Geometry check sheet. Reference: the model listing, model coordinates, mm. Face numbers are marked on the shaded views. A direction names the side the tool comes from. Give positions to 0.01 mm unless a question says otherwise; leave off trailing zeros. Write each loop counter-clockwise with the first axis right and the second up, starting at its lowest first coordinate (ties: lowest second). Pieces come first, ordered by that corner, then holes. Notation, with made-up numbers: (21.25, 82.25) -> (55.25, 82.25) arc R30 cw to (55.25, 113.25) -> close; hole circle Ø2 at (88.5, 82). An arc over 180 degrees is marked (long way). Write item = value, one per line. Start each with the question number.
1. Depth check by flat-ended pin: P1, Ø3, axis at x = -1, z = 14, coming from the +Y side; P2, Ø8, axis at y = 6.5, z = 1.5, coming from the +X side; P3, Ø1.2, axis at x = -0.5, z = -14.5, coming from the -Y side. Enter the tip coordinate at first touch or a pass-through.
2. Cross-section at B-B, the plane y = -19.5. Record the cut outline in (x, z).
3. Cross-section at C-C, the plane z = 14. Record the cut outline in (x, y), plus the area to 3 significant figures.
4. Cross-section at A-A, the plane y = 8. Record the cut outline in (x, z), plus the area to 3 significant figures.
5. Cross-section at D-D, the plane y = 13. Record the cut outline in (x, z).
6. Thickness scan on line 1 along Z through (x, y) = (-1, -19); line 2 along X through (y, z) = (-20.7, -14); line 3 along X through (y, z) = (13, -24). Record the ranges inside material, lowest first.
7. Set-up check for the marked faces 5, 6 and 7: record each of +Z, -Z, +X, -X, +Y, -Y from which the full face is reachable in a straight line by a thin tool's end or side.
8. Mould release check, pull along Z, two halves, no side actions. Record for the marked faces 1, 2, 3 and 4: pulls with the +Z half, pulls with the -Z half, needs draft (parallel to the pull), parting line crosses it, or undercut.
Solid Edge part; units mm, degrees
sketch "Sketch1" plane through (0, 0, 0) normal (1, 0, 0) x (0, 1, 0)
  line L0 (-23.5, -27) -> (23.5, -27)
  line L1 (23.5, -27) -> (23.5, 27)
  line L2 (23.5, 27) -> (-23.5, 27)
  line L3 (-23.5, 27) -> (-23.5, -27)
  dimension "D1" = 23.5
  dimension "D2" = 23.5
extrude "Protrusion1" add sketch "Sketch1" along normal mid plane 12
hole "Bohrung_1" at (-1, -23.5, 14) direction (0, 1, 0) diameter 4 depth 6
hole "Hole1" at (-1, -23.5, -14) direction (0, 1, 0) diameter 4 depth 6
sketch "Sketch2" plane through (6, 0, 0) normal (1, 0, 0) x (0, 1, 0)
  line L0 (23.5, -4) -> (10, 13)
  line L1 (10, 13) -> (10, 3)
  line L2 (10, 3) -> (2.5, 3)
  line L3 (2.5, 3) -> (2.5, 18)
  line L4 (2.5, 18) -> (23.5, 18)
  line L5 (23.5, 18) -> (23.5, -4)
  dimension "D1" = 2.5
  dimension "D2" = 10
  dimension "D3" = 2.5
  dimension "D4" = 10
extrude "Extrusionsausschnitt_1" cut sketch "Sketch2" against normal blind 135.5146
sketch "Sketch3" plane through (6, 0, 0) normal (1, 0, 0) x (0, 1, 0)
  spline S0 degree 3 poles (12.1174, 10.3337) (10.891, 11.9811) (10.2801, 12.3852) (10, 11.2459) knots 0 0 0 0 1 1 1 1
  line L0 (9.0244, 13.5703) -> (10, 11.2459)
  line L1 (12.1174, 14.0202) -> (9.0244, 13.5703)
  line L2 (12.1174, 10.3337) -> (12.1174, 14.0202)
extrude "Extrusionsausschnitt_3" cut sketch "Sketch3" along normal mid plane 89.7467
fillet "Verrundung_1" radius 10 1 edges at (0, 23.5, -4)
sketch "Sketch4" plane through (6, 0, 0) normal (1, 0, 0) x (0, 1, 0)
  line L0 (-23.5, -27) -> (23.5, -27)
  line L1 (23.5, -27) -> (23.5, -25)
  line L2 (23.5, -25) -> (-23.5, -25)
  line L3 (-23.5, -25) -> (-23.5, -27)
  dimension "D1" = 23.5
extrude "Extrusionsausprägung_5" add sketch "Sketch4" along normal blind 2
properties part number "40" material "Polyacticacid"
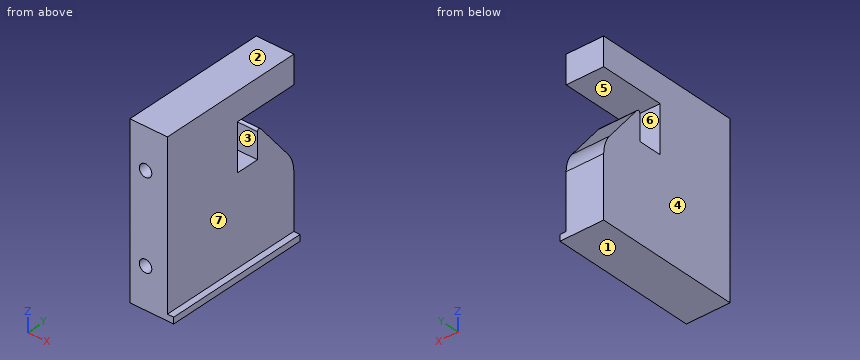
Answers:
q1.P1 = 2.5
q1.P2 = 6
q1.P3 = -17.5
q2.outline = (-6, -27) -> (8, -27) -> (8, -25) -> (6, -25) -> (6, 27) -> (-6, 27) -> close; hole circle Ø4 at (-1, -14); hole circle Ø4 at (-1, 14)
q3.outline = (-6, -23.5) -> (-3, -23.5) -> (-3, -17.5) -> (1, -17.5) -> (1, -23.5) -> (6, -23.5) -> (6, 2.5) -> (-6, 2.5) -> close
q3.area = 288 mm^2
q4.outline = (-6, -27) -> (8, -27) -> (8, -25) -> (6, -25) -> (6, 3) -> (-6, 3) -> close; (-6, 18) -> (6, 18) -> (6, 27) -> (-6, 27) -> close
q4.area = 472 mm^2
q5.outline = (-6, -27) -> (8, -27) -> (8, -25) -> (6, -25) -> (6, 9.22) -> (-6, 9.22) -> close; (-6, 18) -> (6, 18) -> (6, 27) -> (-6, 27) -> close
q6.line_1 = -27 to -16, -12 to 12, 16 to 27
q6.line_2 = -6 to -3, 1 to 6
q6.line_3 = -6 to 6
q7.face_5 = +X, -X, +Y
q7.face_6 = +X, -X
q7.face_7 = +Z, +X, +Y, -Y
q8.face_1 = pulls with the -Z half
q8.face_2 = pulls with the +Z half
q8.face_3 = undercut
q8.face_4 = needs draft
